from build123d import *

# Parameters (mm, degrees)
F0_R     = 1
F1_DEPTH = 5


with BuildPart() as f1:
    # F0 (on Top) → F1 (new body)
    with BuildSketch(Plane.XY):
        with BuildLine():
            add(Edge.make_bspline(
                [(7.693045, 0.489857), (7.064082, 9.124408), (6.435119, 17.758959), (5.806156, 26.39351)],
                knots=[0, 0, 0, 0, 25.972286, 25.972286, 25.972286, 25.972286], degree=3))
            Line((7.693045, 0.489857), (11.638039, 4.607475))
            Line((11.638039, 4.607475), (10.839293, 5.28573))
            Line((10.839293, 5.28573), (11.760553, 6.370649))
            Line((11.760553, 6.370649), (10.722407, 7.252192))
            Line((10.722407, 7.252192), (11.638039, 8.330484))
            Line((11.638039, 8.330484), (10.581676, 9.227495))
            Line((10.581676, 9.227495), (11.471978, 10.275956))
            Line((11.471978, 10.275956), (10.435367, 11.156196))
            Line((10.435367, 11.156196), (11.443965, 12.343969))
            Line((11.443965, 12.343969), (10.32334, 13.295549))
            Line((10.32334, 13.295549), (11.154807, 14.274724))
            Line((11.154807, 14.274724), (10.050478, 15.66664))
            Line((10.050478, 15.66664), (11.568329, 17.454133))
            Line((11.568329, 17.454133), (13.063904, 16.184165))
            Line((13.063904, 16.184165), (12.202819, 15.170112))
            Line((12.202819, 15.170112), (13.257269, 14.274724))
            Line((13.257269, 14.274724), (12.345023, 13.200421))
            Line((12.345023, 13.200421), (13.353622, 12.343969))
            Line((13.353622, 12.343969), (12.345023, 11.156196))
            Line((12.345023, 11.156196), (13.381635, 10.275956))
            Line((13.381635, 10.275956), (12.491333, 9.227495))
            Line((12.491333, 9.227495), (13.547695, 8.330484))
            Line((13.547695, 8.330484), (12.632063, 7.252192))
            Line((12.632063, 7.252192), (13.67021, 6.370649))
            Line((13.67021, 6.370649), (13.197073, 5.813461))
            Line((13.197073, 5.813461), (12.770227, 5.28573))
            add(Edge.make_bspline(
                [(13.769604, 4.466838), (13.436479, 4.739802), (13.103353, 5.012766), (12.770227, 5.28573)],
                knots=[0, 0, 0, 0, 1.292029, 1.292029, 1.292029, 1.292029], degree=3))
            add(Edge.make_bspline(
                [(14.934251, 5.813461), (14.546035, 5.364587), (14.15782, 4.915712), (13.769604, 4.466838)],
                knots=[0, 0, 0, 0, 1.780392, 1.780392, 1.780392, 1.780392], degree=3))
            add(Edge.make_bspline(
                [(13.289604, 23.814345), (13.83782, 17.81405), (14.386036, 11.813755), (14.934251, 5.813461)],
                knots=[0, 0, 0, 0, 18.075859, 18.075859, 18.075859, 18.075859], degree=3))
            add(Edge.make_bspline(
                [(17.661029, 32.037817), (16.203888, 29.29666), (14.746746, 26.555502), (13.289604, 23.814345)],
                knots=[0, 0, 0, 0, 9.313155, 9.313155, 9.313155, 9.313155], degree=3))
            add(Edge.make_bspline(
                [(12.770227, 29.311087), (14.400495, 30.219997), (16.030762, 31.128907), (17.661029, 32.037817)],
                knots=[0, 0, 0, 0, 5.599554, 5.599554, 5.599554, 5.599554], degree=3))
            add(Edge.make_bspline(
                [(10.531368, 44.142015), (11.277654, 39.198373), (12.023941, 34.25473), (12.770227, 29.311087)],
                knots=[0, 0, 0, 0, 14.998964, 14.998964, 14.998964, 14.998964], degree=3))
            add(Edge.make_bspline(
                [(12.2857, 46.500597), (11.653371, 45.717337), (11.021041, 44.934078), (10.531368, 44.142015)],
                knots=[2.939488, 2.939488, 2.939488, 2.939488, 5.878976, 5.878976, 5.878976, 5.878976], degree=3))
            Line((12.2857, 46.500597), (14.040033, 48.859179))
            add(Edge.make_bspline(
                [(9.96209, 46.84221), (11.217791, 47.44206), (12.906654, 48.222175), (14.040033, 48.859179)],
                knots=[1.635184, 1.635184, 1.635184, 1.635184, 5.888303, 5.888303, 5.888303, 5.888303], degree=3))
            Line((9.96209, 46.84221), (8.762033, 46.248656))
            add(Edge.make_bspline(
                [(3.484468, 48.358951), (5.243656, 47.655519), (7.002845, 46.952087), (8.762033, 46.248656)],
                knots=[0, 0, 0, 0, 5.68384, 5.68384, 5.68384, 5.68384], degree=3))
            add(Edge.make_bspline(
                [(7.285437, 44.142015), (6.018447, 45.54766), (4.751458, 46.953306), (3.484468, 48.358951)],
                knots=[0, 0, 0, 0, 5.677139, 5.677139, 5.677139, 5.677139], degree=3))
            add(Edge.make_bspline(
                [(6.060782, 33.975713), (6.469, 37.36448), (6.877219, 40.753248), (7.285437, 44.142015)],
                knots=[0, 0, 0, 0, 10.239799, 10.239799, 10.239799, 10.239799], degree=3))
            add(Edge.make_bspline(
                [(1.129528, 30.918069), (2.773279, 31.937284), (4.417031, 32.956498), (6.060782, 33.975713)],
                knots=[0, 0, 0, 0, 5.80228, 5.80228, 5.80228, 5.80228], degree=3))
            add(Edge.make_bspline(
                [(5.806156, 26.39351), (4.24728, 27.901697), (2.688404, 29.409883), (1.129528, 30.918069)],
                knots=[0, 0, 0, 0, 6.50711, 6.50711, 6.50711, 6.50711], degree=3))
        make_face()
        with Locations((8.249205, 18.715588)):
            Circle(F0_R, mode=Mode.SUBTRACT)
        with BuildLine():
            add(Edge.make_bspline(
                [(8.762033, 46.248656), (9.060568, 46.40761), (9.479315, 46.611587), (9.96209, 46.84221)],
                knots=[0, 0, 0, 0, 1.635184, 1.635184, 1.635184, 1.635184], degree=3))
            Line((8.762033, 46.248656), (9.96209, 46.84221))
        make_face()
        with BuildLine():
            Line((14.040033, 48.859179), (9.96209, 46.84221))
            add(Edge.make_bspline(
                [(9.96209, 46.84221), (11.217791, 47.44206), (12.906654, 48.222175), (14.040033, 48.859179)],
                knots=[1.635184, 1.635184, 1.635184, 1.635184, 5.888303, 5.888303, 5.888303, 5.888303], degree=3))
        make_face()
        with BuildLine():
            add(Edge.make_bspline(
                [(14.040033, 48.859179), (13.550359, 48.067116), (12.91803, 47.283857), (12.2857, 46.500597)],
                knots=[0, 0, 0, 0, 2.939488, 2.939488, 2.939488, 2.939488], degree=3))
            Line((14.040033, 48.859179), (12.2857, 46.500597))
        make_face()
        with BuildLine():
            Line((10.531368, 44.142015), (12.2857, 46.500597))
            add(Edge.make_bspline(
                [(12.2857, 46.500597), (11.653371, 45.717337), (11.021041, 44.934078), (10.531368, 44.142015)],
                knots=[2.939488, 2.939488, 2.939488, 2.939488, 5.878976, 5.878976, 5.878976, 5.878976], degree=3))
        make_face()
    extrude(amount=F1_DEPTH)


solid = f1.part
CAD build for the part. Positions are in the model's coordinates, mm. Give positions to 0.01 mm unless a question says otherwise; leave off trailing zeros. One line per question, with ' | ' between items. Start each with the question number.
1. Probe L1, parallel to X at y = 12, z = 0.3; L2, parallel to X at y = 16, z = 3.8; L3, parallel to X at y = 32.5, z = 4.45. List the from-to ranges inside material, lowest first. Write a range as from..to.
2. Flat gauge pins, fed straight in: pin 1 (3 mm diameter, centred on x = 10, z = 3, fed in from -Y); pin 2 (1.8 mm diameter, centred on x = 8.25, y = 18.72, fed in from -Z); pin 3 (1 mm diameter, centred on x = 12.5, z = 3.5, fed in from +Y); pin 4 (1 mm diameter, centred on x = 5.5, z = 2.5, fed in from +Y). Where does each tip first touch, or does it go through?
3. Two-plate mould, pull along X, no slides. Class faces 1 (the face through (10, 25, 0)), 2 (the face through (10.96, 10.71, 2.46)), 3 (the face through (11.396, 45.305, 2.465)): pulls with the +X half, pulls with the -X half, needs draft (parallel to the pull), parting line crosses it, or undercut.
Result sheet:
1) L1: x = 6.85..11.15, 13.06..14.37 | L2: x = 6.56..10.33, 12.91..14 | L3: x = 3.68..12.29
2) pin 1: stops at y = 1.33 | pin 2: passes through | pin 3: stops at y = 48.34 | pin 4: stops at y = 47.75
3) face 1: needs draft | face 2: undercut | face 3: pulls with the +X half
